Check sheet for the modelled part. Datum: model origin and axes. Units: mm. Coordinates: 2 decimals unless noted, no trailing zeros. Order: outer loops, then holes, each group sorted by start corner. A loop starts at its lowest first (then second) coordinate and runs counter-clockwise, first axis right, second up.
1. Cross-section at A-A (y = -25.4). Enter the section's corners in (x, z), then the cut area to 3 significant figures.
2. Cross-section at C-C (z = 63.5). Enter the section's corners in (x, y), then the cut area to 3 significant figures.
3. Cross-section at B-B (z = 19.05). Enter the section's corners in (x, y).
4. Thickness scan on line 1 (Z direction, x = -1, y = -25.4); line 2 (Z direction, x = 0.8, y = 44.45); line 3 (Y direction, x = 1.4, z = -31.5). Record the ranges inside material, lowest first.
```python
from build123d import *

# Parameters (mm, degrees)
F0_W     = 3.175
F0_H     = 101.6
F1_DEPTH = 69.85
F2_R     = 2.413
F3_DEPTH = 3.175
F4_R     = 2.413
F5_DEPTH = 3.175
F6_R     = 2.413
F7_DEPTH = 3.175
F8_R     = 2.413
F9_DEPTH = 3.175


with BuildPart() as f1:
    # F0 (on Top) → F1 (new body, symmetric)
    with BuildSketch(Plane.XY):
        Rectangle(F0_W, F0_H)
    extrude(amount=F1_DEPTH, both=True)

    # F2 (on face) → F3 (cut, through all)
    with BuildSketch(Plane(origin=(-1.5875, 0, 0), x_dir=(0, -1, 0), z_dir=(-1, 0, 0))):
        with Locations((-44.45, -19.05)):
            Circle(F2_R)
        with Locations((-44.45, 19.05)):
            Circle(F2_R)
    extrude(amount=-F3_DEPTH, mode=Mode.SUBTRACT)

    # F4 (on face) → F5 (cut, through all)
    with BuildSketch(Plane(origin=(-1.5875, 0, 0), x_dir=(0, -1, 0), z_dir=(-1, 0, 0))):
        with Locations((-19.05, -63.5)):
            Circle(F4_R)
        with Locations((-19.05, 63.5)):
            Circle(F4_R)
    extrude(amount=-F5_DEPTH, mode=Mode.SUBTRACT)

    # F6 (on face) → F7 (cut, through all)
    with BuildSketch(Plane(origin=(-1.5875, 0, 0), x_dir=(0, -1, 0), z_dir=(-1, 0, 0))):
        with Locations((25.4, -63.5)):
            Circle(F6_R)
        with Locations((25.4, 63.5)):
            Circle(F6_R)
    extrude(amount=-F7_DEPTH, mode=Mode.SUBTRACT)

    # F8 (on face) → F9 (cut, through all)
    with BuildSketch(Plane.YZ.offset(1.5875)):
        with Locations((-41.402, 31.75)):
            Circle(F8_R)
        with Locations((-41.402, -31.75)):
            Circle(F8_R)
    extrude(amount=-F9_DEPTH, mode=Mode.SUBTRACT)


solid = f1.part
```
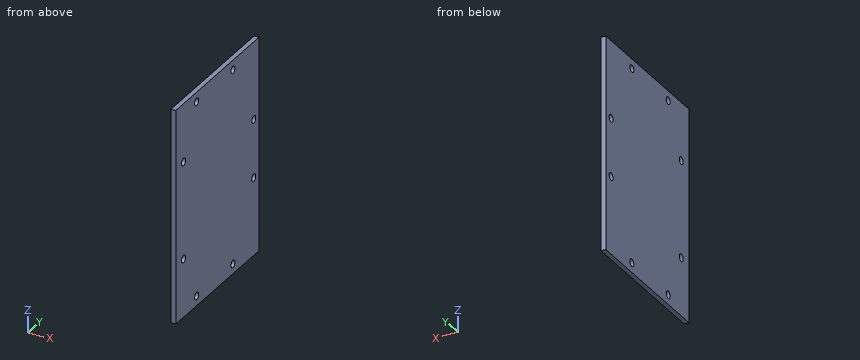
Data:
1. outline: (-1.59, -69.85) - (1.59, -69.85) - (1.59, -65.91) - (-1.59, -65.91) - close; (-1.59, -61.09) - (1.59, -61.09) - (1.59, 61.09) - (-1.59, 61.09) - close; (-1.59, 65.91) - (1.59, 65.91) - (1.59, 69.85) - (-1.59, 69.85) - close
1. area: 413 mm2
2. outline: (-1.59, -50.8) - (1.59, -50.8) - (1.59, -27.81) - (-1.59, -27.81) - close; (-1.59, -22.99) - (1.59, -22.99) - (1.59, 16.64) - (-1.59, 16.64) - close; (-1.59, 21.46) - (1.59, 21.46) - (1.59, 50.8) - (-1.59, 50.8) - close
2. area: 292 mm2
3. outline: (-1.59, -50.8) - (1.59, -50.8) - (1.59, 42.04) - (-1.59, 42.04) - close; (-1.59, 46.86) - (1.59, 46.86) - (1.59, 50.8) - (-1.59, 50.8) - close
4. line 1: z = -69.85 to -65.91, -61.09 to 61.09, 65.91 to 69.85
4. line 2: z = -69.85 to -21.46, -16.64 to 16.64, 21.46 to 69.85
4. line 3: y = -50.8 to -43.8, -39 to 50.8
